from build123d import *
from build123d.topology import SkipClean

# Parameters (mm, degrees)
SKETCH_1_R             = 0.75
EXTRUDE_1_DEPTH        = 2
SKETCH_2_R             = 0.8
SKETCH_4_R             = 1
EXTRUDE_2_DEPTH        = 1.5
SKETCH_5_W             = 9.9
SKETCH_5_H             = 5
EXTRUDE_3_DEPTH        = 4
SKETCH_8_R             = 0.4
EXTRUDE_5_DEPTH        = 2
EXTRUDE_5_2_DEPTH      = 2
SKETCH_9_W             = 2.7
SKETCH_9_H             = 1.8
EXTRUDE_6_DEPTH        = 4
EXTRUDE_4_DEPTH        = 6
SKETCH_7_R             = 1.25
CUT_EXTRUDE_1_DEPTH    = 6
PATTERN_LINEAR_1_COUNT = 2
PATTERN_LINEAR_1_PITCH = 5
CUT_EXTRUDE_START      = -6
CUT_EXTRUDE_2_DEPTH    = 6
FILLET_1_R             = 0.5
FILLET_2_R             = 0.5
FILLET_3_R             = 0.5


with BuildPart() as part:
    # Sketch 1 → Extrude 1 (new body)
    with BuildSketch(Plane.XY):
        Circle(SKETCH_1_R)
    extrude_1 = extrude(amount=-EXTRUDE_1_DEPTH)

    # Sweep 1: sweep along a path in Sketch 3
    with BuildLine(Plane(origin=(0, 0, 0), x_dir=(0, 0, -1), z_dir=(1, 0, 0))) as sweep_1_path:
        ThreePointArc((0, 0), (-1.838477631, 0.761522369), (-2.6, 2.6))
    # Sketch 2 → Sweep 1 (sweep)
    with BuildSketch(Plane.XY):
        Circle(SKETCH_2_R)
    sweep_1 = sweep(path=sweep_1_path.line)

    # Sketch 4 → Extrude 2 (add)
    with BuildSketch(Plane(origin=(0, 2.6, 0), x_dir=(1, 0, 0), z_dir=(0, 1, 0))):
        with Locations(Location((0, -2.6, 0), (0, 0, 270))):
            Circle(SKETCH_4_R)
    extrude_2 = extrude(amount=EXTRUDE_2_DEPTH)

    # Sketch 5 → Extrude 3 (add)
    with BuildSketch(Plane(origin=(0, 4.1, 0), x_dir=(1, 0, 0), z_dir=(0, 1, 0))):
        with Locations((2.5, -2.6)):
            Rectangle(SKETCH_5_W, SKETCH_5_H)
    extrude(amount=EXTRUDE_3_DEPTH)



with BuildPart() as body_2:
    # Sketch 8 → Extrude 5 (new body)
    with BuildSketch(Plane.XY):
        with Locations((-3, 5)):
            Circle(SKETCH_8_R)
    extrude(amount=-EXTRUDE_5_DEPTH)


with BuildPart() as body_3:
    # Sketch 8 → Extrude 5 2 (new body)
    with BuildSketch(Plane.XY):
        with Locations((8, 5)):
            Circle(SKETCH_8_R)
    extrude(amount=-EXTRUDE_5_2_DEPTH)


with BuildPart() as part_1:
    add(part.part)

    add(body_2.part)  # Extrude 6 merges body 2

    add(body_3.part)  # Extrude 6 merges body 3
    # Sketch 9 → Extrude 6 (add)
    with BuildSketch(Plane.XY):
        with Locations((-2.8, 5)):
            Rectangle(SKETCH_9_W, SKETCH_9_H)
        with Locations((7.8, 5)):
            Rectangle(SKETCH_9_W, SKETCH_9_H)
    extrude(amount=EXTRUDE_6_DEPTH)

    # Sketch 6 → Extrude 4 (add)
    with BuildSketch(Plane(origin=(0, 8.1, 0), x_dir=(1, 0, 0), z_dir=(0, 1, 0))):
        with BuildLine():
            Line((0, -0.6), (7, -0.6))
            Line((7, -0.6), (7, -4.6))
            Line((7, -4.6), (0, -4.6))
            ThreePointArc((0, -4.6), (-2, -2.6), (0, -0.6))
        make_face()
    extrude(amount=EXTRUDE_4_DEPTH)

    # Sketch 7 → Cut-Extrude 1 (cut)
    with BuildSketch(Plane(origin=(0, 14.1, 0), x_dir=(1, 0, 0), z_dir=(0, 1, 0))):
        with Locations(Location((0, -2.6, 0), (0, 0, 270))):
            Circle(SKETCH_7_R)
    cut_extrude_1 = extrude(amount=-CUT_EXTRUDE_1_DEPTH, mode=Mode.SUBTRACT)

    # Pattern Linear 1: Extrude 1, Sweep 1, Extrude 2, Cut-Extrude 1 ×2
    with Locations(*[(i * PATTERN_LINEAR_1_PITCH, 0, 0) for i in range(1, PATTERN_LINEAR_1_COUNT)]):
        add(extrude_1)
        add(sweep_1)
        add(extrude_2)
        add(cut_extrude_1, mode=Mode.SUBTRACT)

    # Sketch 10 → Cut-Extrude 2 (cut)
    with SkipClean():  # the faces are left unmerged after this step: merging them gives an invalid solid
        with BuildSketch(Plane(origin=(0, 14.1, 0), x_dir=(1, 0, 0), z_dir=(0, 1, 0)).offset(CUT_EXTRUDE_START)):
            with BuildLine():
                Line((0, -0.6), (5, -0.6))
                ThreePointArc((5, -0.6), (3.971008489, -0.885014149), (3.235294118, -1.658823529))
                ThreePointArc((3.235294118, -1.658823529), (2.5, -2.1), (1.764705882, -1.658823529))
                ThreePointArc((1.764705882, -1.658823529), (1.028991511, -0.885014149), (0, -0.6))
            make_face()
        cut_extrude_2 = extrude(amount=CUT_EXTRUDE_2_DEPTH, mode=Mode.SUBTRACT)

    # Mirror 1: Cut-Extrude 2 across plane
    with SkipClean():  # the faces are left unmerged after this step: merging them gives an invalid solid
        add(cut_extrude_2.mirror(Plane.XY.offset(2.6)), mode=Mode.SUBTRACT)

    # Fillet 1
    fillet_1_edges = [part_1.edges().sort_by_distance(p)[0] for p in [
        (-4.15, 4.1, 2),
        (-4.15, 5.9, 2),
        (9.15, 5.9, 2),
        (9.15, 4.1, 2),
    ]]
    fillet(fillet_1_edges, radius=FILLET_1_R)

    # Fillet 2
    fillet_2_edges = [part_1.edges().sort_by_distance(p)[0] for p in [
        (7.45, 7, 0.1),
        (-2.45, 7, 0.1),
        (-2.45, 6.1, 5.1),
        (7.45, 6.1, 5.1),
    ]]
    fillet(fillet_2_edges, radius=FILLET_2_R)

    # Fillet 3
    fillet_3_edges = [part_1.edges().sort_by_distance(p)[0] for p in [
        (7, 11.1, 4.6),
        (7, 11.1, 0.6),
    ]]
    fillet(fillet_3_edges, radius=FILLET_3_R)


solid = part_1.part
Input: part model. Units: mm. Frame: model coordinates. A direction names the side the tool comes from. Give positions to 0.01 mm unless a question says otherwise; leave off trailing zeros. Write each loop counter-clockwise with the first axis right and the second up, starting at its lowest first coordinate (ties: lowest second). Pieces come first, ordered by that corner, then holes. Notation, with made-up numbers: M 50,-20.5 L 81,-20.5 A10 cw 81,-15.5 Z; hole C 63,11 d7. An arc over 180 degrees is marked long. Write item = value, one per line. Start each with the question number.
1) Cut plane C-C on y = 8.75. Return the cut outline in (x, z).
2) Cut plane D-D on y = 3.5. Return the cut outline in (x, z), then the cut area to 3 significant figures.
3) Reachability of faces 4 (the cylindrical face through (2.5, 11.1, 3.1)), 5 (the cylindrical face through (-3.295, 5.27, -0.986)), 6 (the flat face through (6, 11, 0.6)), 7 (the cylindrical face through (2.5, 11.1, 2.1)) from +Z, -Z, +X, -X, +Y, -Y: full face, straight path, thin tool, end or side. Return the list, or none.
4) Cut plane B-B on y = 5. Return the cut outline in (x, z).
5) First-contact query: pin 1 Ø1.1 at (x, z) = (-2.5, 1.5) entering from +Y; pin 2 Ø3 at (x, z) = (1.5, 0.5) entering from -Y; pin 3 Ø1.9 at (x, y) = (8.5, 5) entering from +Z; pin 4 Ø1.5 at (y, z) = (9.5, -0.5) entering from -X. Flat tips, straight axial feed; report the tip coordinate or a pass-through.
6) Cut plane A-A on x = 8. Return the cut outline in (y, z), then the cut area to 3 significant figures.
7) Material intervals for line 1 along X through (y, z) = (10.4, 2.6); line 2 along X through (y, z) = (11.5, 3.5); line 3 along Y through (x, z) = (8, 1), sorted ascending. Write a range as [from, to].
8) Draft query along X for faces 1 (the flat face through (-3, 5, 4)), 2 (the flat face through (-4.15, 5, 2)), 3 (the flat face through (2, 8.1, 4)). Return one class per face: +X half, -X half, draft (parallel to the pull), parting line (faces both ways), or undercut.
Solved:
q1.outline = M 1.76,1.66 A0.83 cw 3.24,1.66 A2 ccw 5,0.6 L 6.5,0.6 A0.5 ccw 7,1.1 L 7,4.1 A0.5 ccw 6.5,4.6 L 5,4.6 A2 ccw 3.24,3.54 A0.83 cw 1.76,3.54 A2 ccw long Z; hole C 0,2.6 d2.5; hole C 5,2.6 d2.5
q2.outline = C 0,2.6 d2; C 5,2.6 d2
q2.area = 6.28 mm2
q3.face_4 = +Z, +Y
q3.face_5 = -Z
q3.face_6 = -Z, +X, -X, +Y
q3.face_7 = -Z, +Y
q4.outline = M -4.15,0 L -3.4,0 L -3.4,-2 L -2.6,-2 L -2.6,0 L -1.45,0 L -1.45,0.1 L 6.45,0.1 L 6.45,0 L 7.6,0 L 7.6,-2 L 8.4,-2 L 8.4,0 L 9.15,0 L 9.15,4 L 7.45,4 L 7.45,4.6 A0.5 ccw 6.95,5.1 L -1.95,5.1 A0.5 ccw -2.45,4.6 L -2.45,4 L -4.15,4 Z
q5.pin_1 = 8.1
q5.pin_2 = -0.8
q5.pin_3 = 4
q5.pin_4 = through
q6.outline = M 4.1,0 L 4.6,0 L 4.6,-2 L 5.4,-2 L 5.4,0 L 5.9,0 L 5.9,4 L 4.1,4 Z
q6.area = 8.80 mm2
q7.line_1 = [-2, -1.25], [1.25, 3.75], [6.25, 7]
q7.line_2 = [-1.79, -0.87], [0.87, 1.79], [3.21, 4.13], [5.87, 7]
q7.line_3 = [4.1, 5.9]
q8.face_1 = draft
q8.face_2 = -X half
q8.face_3 = undercut
